Verification items for the finished model (mm, model axes). Face numbers are marked on the shaded views. Round coordinates to 2 decimals unless told otherwise and drop trailing zeros. Loops run counter-clockwise (first coordinate to the right, second up) from the corner with the lowest first, then second, coordinate; pieces in that order, holes last. Notation, with made-up numbers: M 31,59 L 75,59 A10 cw 75,66 Z; hole C 23,73 d7. An arc over 180 degrees is marked long. One line per item, written item: value.
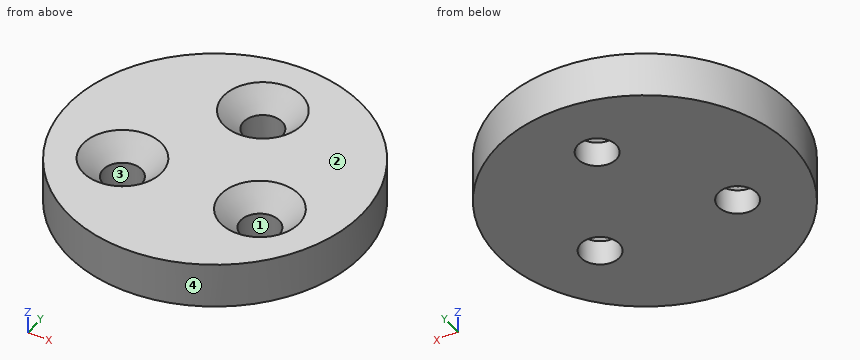
from build123d import *

# Parameters (mm, degrees)
SKETCH1_R                                            = 13
BOSS_EXTRUDE1_DEPTH                                  = 4
CSK_FOR_M3_HEX_SOCKET_COUNTERSUNK_HEAD_S_D           = 3.4
CSK_FOR_M3_HEX_SOCKET_COUNTERSUNK_HEAD_S_DEPTH       = 12
CSK_FOR_M3_HEX_SOCKET_COUNTERSUNK_HEAD_S_CSINK_D     = 6.94
CSK_FOR_M3_HEX_SOCKET_COUNTERSUNK_HEAD_S_CSINK_ANGLE = 90
CSK_FOR_M3_HEX_SOCKET_COUNTERSUNK_HEAD_S_TIP         = 1.021463052


with BuildPart() as part:
    # Sketch1 → Boss-Extrude1 (new body)
    with BuildSketch(Plane.XY):
        Circle(SKETCH1_R)
    extrude(amount=BOSS_EXTRUDE1_DEPTH)

    # CSK for M3 Hex Socket Countersunk Head Screw1
    with Locations(Plane.XY.offset(4)):
        with Locations((0, 7), (6.062177826, -3.5), (-6.062177826, -3.5)):
            CounterSinkHole(CSK_FOR_M3_HEX_SOCKET_COUNTERSUNK_HEAD_S_D / 2, CSK_FOR_M3_HEX_SOCKET_COUNTERSUNK_HEAD_S_CSINK_D / 2, depth=CSK_FOR_M3_HEX_SOCKET_COUNTERSUNK_HEAD_S_DEPTH, counter_sink_angle=CSK_FOR_M3_HEX_SOCKET_COUNTERSUNK_HEAD_S_CSINK_ANGLE)
            with Locations((0, 0, -(CSK_FOR_M3_HEX_SOCKET_COUNTERSUNK_HEAD_S_DEPTH + CSK_FOR_M3_HEX_SOCKET_COUNTERSUNK_HEAD_S_TIP / 2))):  # 118° drill point
                Cone(0, CSK_FOR_M3_HEX_SOCKET_COUNTERSUNK_HEAD_S_D / 2, CSK_FOR_M3_HEX_SOCKET_COUNTERSUNK_HEAD_S_TIP, mode=Mode.SUBTRACT)


solid = part.part
(1) Sectioned sample at A-A on x = 0. Enter the section's corners in (y, z), and give its area (3 significant figures).
Completed:
outline: M -13,0 L 5.3,0 L 5.3,2.23 L 3.53,4 L -13,4 Z; M 8.7,0 L 13,0 L 13,4 L 10.47,4 L 8.7,2.23 Z
area: 87.3 mm^2
(2) Mould release check, pull along Y, two halves, no side actions. Record for the marked faces 1, 2, 3 and 4: +Y half, -Y half, draft (parallel to the pull), parting line (faces both ways), or undercut.
Completed:
face 1: undercut
face 2: draft
face 3: undercut
face 4: parting line
(3) Sectioned sample at B-B on y = -3.5. Enter the section's corners in (x, z), and give its area (3 significant figures).
Completed:
outline: M -12.52,0 L -7.76,0 L -7.76,2.23 L -9.53,4 L -12.52,4 Z; M -4.36,0 L 4.36,0 L 4.36,2.23 L 2.59,4 L -2.59,4 L -4.36,2.23 Z; M 7.76,0 L 12.52,0 L 12.52,4 L 9.53,4 L 7.76,2.23 Z
area: 66.7 mm^2
(4) Depth check by flat-ended pin: pin 1 Ø1.5 at (x, z) = (6, 3) entering from +Y; pin 2 Ø2.5 at (x, y) = (6.06, -3.5) entering from +Z. Enter the tip coordinate at first touch or a pass-through.
Completed:
pin 1: stops at y = 11.89
pin 2: passes through
(5) Thickness scan on L1, parallel to X at y = -3.5, z = 0.95; L2, parallel to Y at x = 0, z = 0.75; L3, parallel to Y at x = 7, z = 0.95. Record the ranges inside material, lowest first. Write a range as from..to.
Completed:
L1: x = -12.52..-7.76, -4.36..4.36, 7.76..12.52
L2: y = -13..5.3, 8.7..13
L3: y = -10.95..-4.92, -2.08..10.95
(6) Sectioned sample at D-D on z = 1.15. Enter the section's corners in (x, y), and give its area (3 significant figures).
Completed:
outline: C 0,0 d26; hole C -6.06,-3.5 d3.4; hole C 0,7 d3.4; hole C 6.06,-3.5 d3.4
area: 504 mm^2
(7) Sectioned sample at C-C on y = 7. Enter the section's corners in (x, z).
Completed:
outline: M -10.95,0 L -1.7,0 L -1.7,2.23 L -3.47,4 L -10.95,4 Z; M 1.7,0 L 10.95,0 L 10.95,4 L 3.47,4 L 1.7,2.23 Z
